Model file for the job. Use its own axes, mm. Face numbers are marked on the shaded views. A direction names the side the tool comes from. Coordinates: 2 decimals unless noted, no trailing zeros. Order: outer loops, then holes, each group sorted by start corner. A loop starts at its lowest first (then second) coordinate and runs counter-clockwise, first axis right, second up.
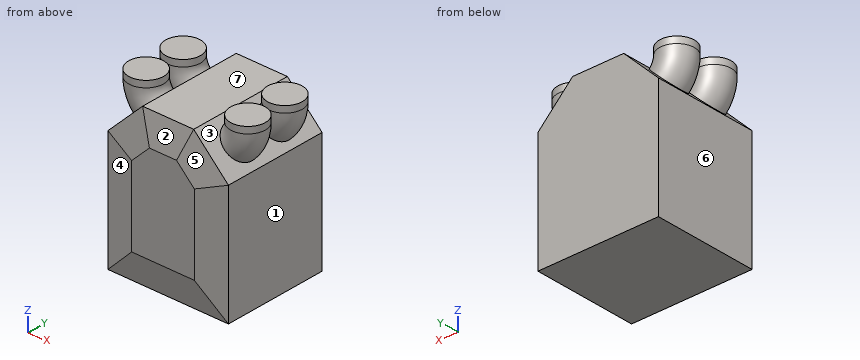
from build123d import *

# Parameters (mm, degrees)
F0_W     = 625
F0_H     = 801
F1_DEPTH = 572
F2_SIZE  = 180
F4_R     = 90
F8_SIZE2 = 30
F8_SIZE  = 150


with BuildPart() as f1:
    # F0 (on Front) → F1 (new body)
    with BuildSketch(Plane.XZ):
        with Locations((0, 400.5)):
            Rectangle(F0_W, F0_H)
    extrude(amount=F1_DEPTH)

    # F2
    f2_edges = [f1.edges().sort_by_distance(p)[0] for p in [
        (-312.5, -286, 801),
        (312.5, -286, 801),
    ]]
    chamfer(f2_edges, length=F2_SIZE)

    # F6: sweep along a path in F5
    with BuildLine(Plane(origin=(0, 0, 0), x_dir=(-1, 0, 0), z_dir=(0, 1, 0))) as f6_path:
        Line((-264, 845), (-264, 811.1898628385))
        ThreePointArc((-264, 811.1898628385), (-253.2145014023, 756.9674997961), (-222.5, 711))
    # F4 (on offset) → F6 (sweep)
    with BuildSketch(Plane.XY.offset(845)):
        with Locations((264, -161)):
            Circle(F4_R)
        with Locations((264, -375)):
            Circle(F4_R)
    sweep(path=f6_path.line)

    # F7: sweep along a path in F5
    with BuildLine(Plane(origin=(0, 0, 0), x_dir=(-1, 0, 0), z_dir=(0, 1, 0))) as f7_path:
        Line((264, 845), (264, 811.1898628385))
        ThreePointArc((264, 811.1898628385), (253.2145014023, 756.9674997961), (222.5, 711))
    # F4 (on offset) → F7 (sweep)
    with BuildSketch(Plane.XY.offset(845)):
        with Locations((-264, -375)):
            Circle(F4_R)
        with Locations((-264, -161)):
            Circle(F4_R)
    sweep(path=f7_path.line)

    # F8
    f8_edges = [f1.edges().sort_by_distance(p)[0] for p in [
        (-312.5, -572, 310.5),
        (-222.5, -572, 711),
        (0, -572, 0),
        (0, -572, 801),
        (312.5, -572, 310.5),
        (222.5, -572, 711),
    ]]
    f8_side = f1.faces().sort_by_distance((0, -572, 376.938251))[0]
    chamfer(f8_edges, length=F8_SIZE, length2=F8_SIZE2, reference=f8_side)


solid = f1.part
Q1. Probe line 1 (X direction, y = -336, z = 797.5); line 2 (X direction, y = -302, z = 57.5); line 3 (X direction, y = -371.5, z = 784). List the from-to ranges inside material, lowest first.
Established:
line 1: x = -344.69 to -181.32, -136 to 136, 181.32 to 344.69
line 2: x = -312.5 to 312.5
line 3: x = -352.33 to -166.35, -149.5 to 149.5, 166.35 to 352.33
Q2. Cut at D-D, the plane y = -434.5. List the corners of the cut face in (x, z).
Established:
outline: (-331.53, 811.19) arc R209.22 ccw to (-270.25, 663.25) - (-312.5, 621) - (-312.5, 0) - (312.5, 0) - (312.5, 621) - (270.25, 663.25) arc R209.22 ccw to (331.53, 811.19) - (331.53, 845) - (196.47, 845) - (196.47, 811.19) arc R74.16 cw to (174.75, 758.75) - (132.5, 801) - (-132.5, 801) - (-174.75, 758.75) arc R74.16 cw to (-196.47, 811.19) - (-196.47, 845) - (-331.53, 845) - close
Q3. Which spindle directions (+Z, -Z, +X, -X, +Y, -Y) get a long thin tool onto all of the face, cutting with end or side? Do the marked faces 5, 6 and 7. Say none if no direction does.
Established:
face 5: +Z, +X, -Y
face 6: -Z, -X, +Y, -Y
face 7: +Z, +Y, -Y
Q4. Drop flat-ended pins along their axis: P1, Ø1, axis at x = -156.5, z = 495, coming from the +Y side; P2, Ø1, axis at y = -510.5, z = 258.5, coming from the -X side; P3, Ø1, axis at x = 224, z = 367.5, coming from the -Y side; P4, Ø1.5, axis at x = 36, y = -210, coming from the +Z side. Give the stop position or say it passes through.
Established:
P1: stops at y = 0
P2: stops at x = -312.5
P3: stops at y = -559.8
P4: stops at z = 801
Q5. Cut at B-B, the plane x = -115. List the corners of the cut face in (y, z).
Established:
outline: (-572, 150) - (-542, 0) - (0, 0) - (0, 801) - (-542, 801) - (-550.45, 758.75) - (-572, 606.37) - close
Q6. Mould opens along X. For the marked faces 1, 2, 3 and 4 say: pulls with the +X half, pulls with the -X half, needs draft (parallel to the pull), parting line crosses it, or undercut.
Established:
face 1: pulls with the +X half
face 2: needs draft
face 3: undercut
face 4: pulls with the -X half
Q7. Cut at A-A, the plane y = -263.5. List the corners of the cut face in (x, z).
Established:
outline: (-312.5, 0) - (312.5, 0) - (312.5, 621) - (132.5, 801) - (-132.5, 801) - (-312.5, 621) - close
Q8. Cut at C-C, the plane z = 281. List the corners of the cut face in (x, y), plus the area to 3 significant figures.
Established:
outline: (-312.5, -542) - (-162.5, -572) - (162.5, -572) - (312.5, -542) - (312.5, 0) - (-312.5, 0) - close
area: 353,000 mm2
